```python
from build123d import *

# Parameters (mm, degrees)
SKETCH1_R           = 75
SKETCH1_R_2         = 4.25
BOSS_EXTRUDE1_DEPTH = 6.5
BOSS_EXTRUDE2_DEPTH = 12
CHAMFER1_SIZE       = 2
CUT_EXTRUDE1_START  = -6.5
CUT_EXTRUDE1_DEPTH  = 6.5
SKETCH5_R           = 3.5
CUT_EXTRUDE3_DEPTH  = 6.5
SKETCH4_R           = 4
CUT_EXTRUDE5_DEPTH  = 6.5


with BuildPart() as part:
    # Sketch1 → Boss-Extrude1 (new body)
    with BuildSketch(Plane(origin=(0, 0, 0), x_dir=(1, 0, 0), z_dir=(0, 1, 0))):
        with Locations(Location((0, 0, 0), (0, 0, 90))):
            Circle(SKETCH1_R)
        with Locations(Location((0, 0, 0), (0, 0, 90))):
            Circle(SKETCH1_R_2, mode=Mode.SUBTRACT)
    extrude(amount=BOSS_EXTRUDE1_DEPTH)

    # Sketch2 → Boss-Extrude2 (add)
    with BuildSketch(Plane(origin=(0, 6.5, 0), x_dir=(1, 0, 0), z_dir=(0, 1, 0))):
        with BuildLine():
            Line((-13, -13), (-73.86474125, -13))
            ThreePointArc((-73.86474125, -13), (-73.483557376, -15.005558816), (-73.047929471, -17))
            Line((-73.047929471, -17), (-32, -17))
            ThreePointArc((-32, -17), (-21.393398282, -21.393398282), (-17, -32))
            Line((-17, -32), (-17, -73.047929471))
            ThreePointArc((-17, -73.047929471), (-15.005558816, -73.483557376), (-13, -73.86474125))
            Line((-13, -73.86474125), (-13, -13))
        make_face()
        with BuildLine():
            Line((-32, 17), (-73.047929471, 17))
            ThreePointArc((-73.047929471, 17), (-73.483557376, 15.005558816), (-73.86474125, 13))
            Line((-73.86474125, 13), (-13, 13))
            Line((-13, 13), (-13, 73.86474125))
            ThreePointArc((-13, 73.86474125), (-15.005558816, 73.483557376), (-17, 73.047929471))
            Line((-17, 73.047929471), (-17, 32))
            ThreePointArc((-17, 32), (-21.393398282, 21.393398282), (-32, 17))
        make_face()
        with BuildLine():
            Line((17, 32), (17, 73.047929471))
            ThreePointArc((17, 73.047929471), (15.005558816, 73.483557376), (13, 73.86474125))
            Line((13, 73.86474125), (13, 13))
            Line((13, 13), (73.86474125, 13))
            ThreePointArc((73.86474125, 13), (73.483557376, 15.005558816), (73.047929471, 17))
            Line((73.047929471, 17), (32, 17))
            ThreePointArc((32, 17), (21.393398282, 21.393398282), (17, 32))
        make_face()
        with BuildLine():
            Line((32, -17), (73.047929471, -17))
            ThreePointArc((73.047929471, -17), (73.483557376, -15.005558816), (73.86474125, -13))
            Line((73.86474125, -13), (13, -13))
            Line((13, -13), (13, -73.86474125))
            ThreePointArc((13, -73.86474125), (15.005558816, -73.483557376), (17, -73.047929471))
            Line((17, -73.047929471), (17, -32))
            ThreePointArc((17, -32), (21.393398282, -21.393398282), (32, -17))
        make_face()
    extrude(amount=BOSS_EXTRUDE2_DEPTH)

    # Chamfer1
    chamfer1_edges = [part.edges().sort_by_distance(p)[0] for p in [
        (-13, 12.5, 13),
        (-13, 18.5, 43.432370625),
        (-43.432370625, 18.5, 13),
        (13, 12.5, 13),
        (43.432370625, 18.5, 13),
        (13, 18.5, 43.432370625),
        (-13, 12.5, -13),
        (-43.432370625, 18.5, -13),
        (-13, 18.5, -43.432370625),
        (13, 12.5, -13),
        (13, 18.5, -43.432370625),
        (43.432370625, 18.5, -13),
    ]]
    chamfer(chamfer1_edges, length=CHAMFER1_SIZE)

    # Sketch3 → Cut-Extrude1 (cut)
    with BuildSketch(Plane(origin=(0, 6.5, 0), x_dir=(1, 0, 0), z_dir=(0, 1, 0)).offset(CUT_EXTRUDE1_START)):
        with BuildLine():
            Line((32, -17), (48.083261121, -17))
            ThreePointArc((48.083261121, -17), (36.062445841, -36.062445841), (17, -48.083261121))
            Line((17, -48.083261121), (17, -32))
            ThreePointArc((17, -32), (21.393398282, -21.393398282), (32, -17))
        make_face()
        with BuildLine():
            Line((-17, -32), (-17, -48.083261121))
            ThreePointArc((-17, -48.083261121), (-36.062445841, -36.062445841), (-48.083261121, -17))
            Line((-48.083261121, -17), (-32, -17))
            ThreePointArc((-32, -17), (-21.393398282, -21.393398282), (-17, -32))
        make_face()
        with BuildLine():
            Line((17, 32), (17, 48.083261121))
            ThreePointArc((17, 48.083261121), (36.062445841, 36.062445841), (48.083261121, 17))
            Line((48.083261121, 17), (32, 17))
            ThreePointArc((32, 17), (21.393398282, 21.393398282), (17, 32))
        make_face()
        with BuildLine():
            Line((-32, 17), (-48.083261121, 17))
            ThreePointArc((-48.083261121, 17), (-36.062445841, 36.062445841), (-17, 48.083261121))
            Line((-17, 48.083261121), (-17, 32))
            ThreePointArc((-17, 32), (-21.393398282, 21.393398282), (-32, 17))
        make_face()
    extrude(amount=CUT_EXTRUDE1_DEPTH, mode=Mode.SUBTRACT)

    # Sketch5 → Cut-Extrude3 (cut)
    with BuildSketch(Plane(origin=(0, 6.5, 0), x_dir=(1, 0, 0), z_dir=(0, 1, 0))):
        with Locations(Location((65, 0, 0), (0, 0, 270))):
            Circle(SKETCH5_R)
        with Locations(Location((39, 0, 0), (0, 0, 270))):
            Circle(SKETCH5_R)
        with Locations(Location((-39, 0, 0), (0, 0, 270))):
            Circle(SKETCH5_R)
        with Locations(Location((-65, 0, 0), (0, 0, 270))):
            Circle(SKETCH5_R)
    extrude(amount=-CUT_EXTRUDE3_DEPTH, mode=Mode.SUBTRACT)

    # Sketch4 → Cut-Extrude5 (cut)
    with BuildSketch(Plane(origin=(0, 6.5, 0), x_dir=(1, 0, 0), z_dir=(0, 1, 0))):
        with Locations(Location((44.547727215, -44.547727215, 0), (0, 0, 270))):
            Circle(SKETCH4_R)
        with Locations(Location((-44.547727215, -44.547727215, 0), (0, 0, 270))):
            Circle(SKETCH4_R)
        with Locations(Location((44.547727215, 44.547727215, 0), (0, 0, 270))):
            Circle(SKETCH4_R)
        with Locations(Location((-44.547727215, 44.547727215, 0), (0, 0, 270))):
            Circle(SKETCH4_R)
    extrude(amount=-CUT_EXTRUDE5_DEPTH, mode=Mode.SUBTRACT)


solid = part.part
```
Check sheet for the modelled part. Datum: model origin and axes. Units: mm. A direction names the side the tool comes from. Coordinates: 2 decimals unless noted, no trailing zeros. Order: outer loops, then holes, each group sorted by start corner. A loop starts at its lowest first (then second) coordinate and runs counter-clockwise, first axis right, second up. Notation, with made-up numbers: M 10.25,24 L 61.25,24 A25 ccw 61.25,58 Z; hole C -10.75,8 d3. An arc over 180 degrees is marked long. Write each question's results on one line, items separated by ' | '. Start each with the question number.
1. Go/stop test with flat-tipped pins: P1, Ø11, axis at x = -30.5, y = 13, coming from the +Z side; P2, Ø8, axis at y = 9.5, z = 56, coming from the +X side; P3, Ø8, axis at x = 6, y = 7, coming from the -Z side. Record where each tip stops, or that it passes through.
2. Cross-section at A-A on y = 14.25. State how many separate pieces and enclosed holes the cut face has, and give its area (3 significant figures).
3. Cross-section at B-B on z = 0. Record the cut outline in (x, y), and give its area (3 significant figures).
4. Mould release check, pull along Z, two halves, no side actions. Record for faces 1 (the face through (42.47, 3.3, -0.46)), 2 (the face through (-18, 18.5, -25)): +Z half, -Z half, draft (parallel to the pull), parting line (faces both ways), or undercut.
5. Cross-section at D-D on z = -27. Record the cut outline in (x, y), and give its area (3 significant figures).
6. Access from +Z, -Z, +X, -X, +Y, -Y to the whole of each face (thin tool, end or side, straight path). Record for faces 3 (the face through (17, 11, -52)), 4 (the face through (-13, 11, 45)), 5 (the face through (-45, 6.5, -38)), 6 (the face through (21.51, 9.12, -21.28)).
7. Material ranges on probe 1 along X at (y, z) = (2.75, 0.5); probe 2 along Z at (x, y) = (38.5, 8.25), recorded low to high.
8. Cross-section at C-C on x = 20.5. Record the cut outline in (y, z), and give its area (3 significant figures).
Checks:
1) P1: stops at z = 18.73 | P2: stops at x = 52.71 | P3: stops at z = -74.97
2) separate pieces: 4 | enclosed holes: 0 | area: 2,060 mm²
3) outline: M -75,0 L -68.5,0 L -68.5,6.5 L -75,6.5 Z; M -61.5,0 L -42.5,0 L -42.5,6.5 L -61.5,6.5 Z; M -35.5,0 L -4.25,0 L -4.25,6.5 L -35.5,6.5 Z; M 4.25,0 L 35.5,0 L 35.5,6.5 L 4.25,6.5 Z; M 42.5,0 L 61.5,0 L 61.5,6.5 L 42.5,6.5 Z; M 68.5,0 L 75,0 L 75,6.5 L 68.5,6.5 Z | area: 738 mm²
4) face 1: undercut | face 2: draft
5) outline: M -69.97,0 L -43.27,0 L -43.27,6.5 L -69.97,6.5 Z; M -17.86,0 L 17.86,0 L 17.86,18.5 L 15,18.5 L 13,16.5 L 13,6.5 L -13,6.5 L -13,16.5 L -15,18.5 L -17.86,18.5 Z; M 43.27,0 L 69.97,0 L 69.97,6.5 L 43.27,6.5 Z | area: 692 mm²
6) face 3: +Y | face 4: +Z, -Z, +Y | face 5: -Z, -X, +Y | face 6: +Y, -Y
7) probe 1: x = -75 to -68.46, -61.54 to -42.46, -35.54 to -4.22, 4.22 to 35.54, 42.46 to 61.54, 68.46 to 75 | probe 2: z = -17 to -13, 13 to 17
8) outline: M 0,-72.14 L 6.5,-72.14 L 6.5,-46.7 L 0,-46.7 Z; M 0,-22.37 L 18.5,-22.37 L 18.5,-15 L 16.5,-13 L 6.5,-13 L 6.5,13 L 16.5,13 L 18.5,15 L 18.5,22.37 L 0,22.37 Z; M 0,46.7 L 6.5,46.7 L 6.5,72.14 L 0,72.14 Z | area: 842 mm²
